Source: three-view drawing plus pictorial views. Frame: mm from the lowest corner of the part. A direction names the side the tool comes from. Coordinates: 2 decimals unless noted, no trailing zeros. Loops run counter-clockwise (first coordinate to the right, second up) from the corner with the lowest first, then second, coordinate; pieces in that order, holes last. Notation, with made-up numbers: M 62.5,-1 L 118.5,-1 A29 cw 118.5,38 Z; hole C -36.5,55 d11. An arc over 180 degrees is marked long. Use a Markdown table: item, result. Add a question column.
1. Pin query (flat end, axial travel): pin 1 (1.8 mm diameter, centred on y = 5.2, z = 63, fed in from +X); pin 2 (3.5 mm diameter, centred on x = 51.3, z = 101.25, fed in from -Y). Return the tip coordinate at first contact, or that it passes through.
2. Section A-A on z = 31.5. Output: boundary loops of the cut face in (x, y) (3 decimals), then the cut area to 3 significant figures.
3. Line query: L1, parallel to X at y = 10.75, z = 32; L2, parallel to X at y = 11.3, z = 123.25; L3, parallel to X at y = 3.5, z = 12 (3 decimals). Output: solid intervals per line, ascending. Write a range as [from, to].
4. Section D-D on z = 93.5. Output: boundary loops of the cut face in (x, y) (3 decimals).
5. Section B-B on x = 23. Output: boundary loops of the cut face in (y, z).
6. Set-up query: the marked faces 1 and 2. Return all of +Z, -Z, +X, -X, +Y, -Y with unobstructed straight access to the full face (end or side cutting, diameter ignored); none if empty.
7. Section C-C on z = 49. Output: boundary loops of the cut face in (x, y) (3 decimals).
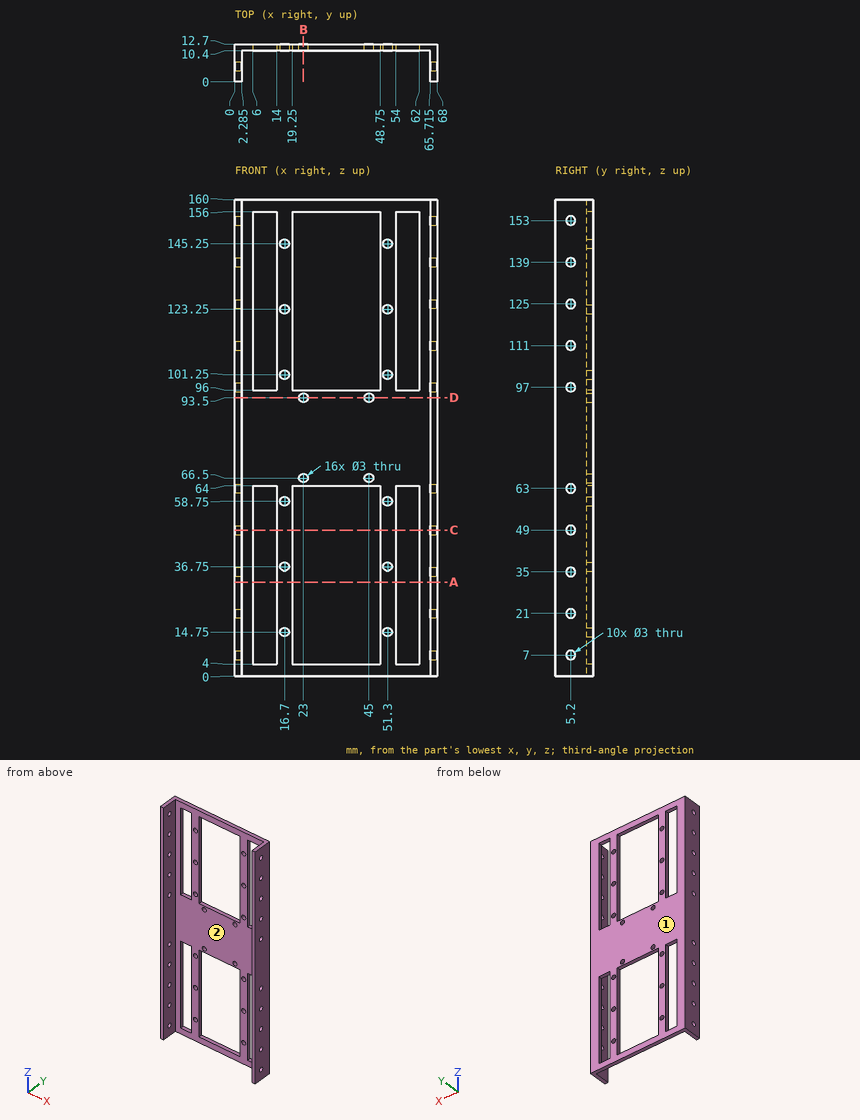
Answers below:
| question | item | result |
|---|---|---|
| 1 | pin 1 | passes through |
| 1 | pin 2 | stops at y = 10.4 |
| 2 | outline | M 0,0 L 2.285,0 L 2.285,10.4 L 6,10.4 L 6,12.7 L 0,12.7 Z; M 14,10.4 L 19.25,10.4 L 19.25,12.7 L 14,12.7 Z; M 48.75,10.4 L 54,10.4 L 54,12.7 L 48.75,12.7 Z; M 62,10.4 L 65.715,10.4 L 65.715,0 L 68,0 L 68,12.7 L 62,12.7 Z |
| 2 | area | 99.3 mm² |
| 3 | L1 | x = [0, 6], [14, 19.25], [48.75, 54], [62, 68] |
| 3 | L2 | x = [0, 6], [14, 15.2], [18.2, 19.25], [48.75, 49.8], [52.8, 54], [62, 68] |
| 3 | L3 | x = [0, 2.285], [65.715, 68] |
| 4 | outline | M 0,0 L 2.285,0 L 2.285,10.4 L 21.5,10.4 L 21.5,12.7 L 0,12.7 Z; M 24.5,10.4 L 43.5,10.4 L 43.5,12.7 L 24.5,12.7 Z; M 46.5,10.4 L 65.715,10.4 L 65.715,0 L 68,0 L 68,12.7 L 46.5,12.7 Z |
| 5 | outline | M 10.4,0 L 12.7,0 L 12.7,4 L 10.4,4 Z; M 10.4,64 L 12.7,64 L 12.7,65 L 10.4,65 Z; M 10.4,68 L 12.7,68 L 12.7,92 L 10.4,92 Z; M 10.4,95 L 12.7,95 L 12.7,96 L 10.4,96 Z; M 10.4,156 L 12.7,156 L 12.7,160 L 10.4,160 Z |
| 6 | face 1 | +Z, -Z, +X, -X, +Y |
| 6 | face 2 | +Z, -Z, -Y |
| 7 | outline | M 0,0 L 2.285,0 L 2.285,3.7 L 0,3.7 Z; M 0,6.7 L 2.285,6.7 L 2.285,10.4 L 6,10.4 L 6,12.7 L 0,12.7 Z; M 14,10.4 L 19.25,10.4 L 19.25,12.7 L 14,12.7 Z; M 48.75,10.4 L 54,10.4 L 54,12.7 L 48.75,12.7 Z; M 62,10.4 L 65.715,10.4 L 65.715,6.7 L 68,6.7 L 68,12.7 L 62,12.7 Z; M 65.715,0 L 68,0 L 68,3.7 L 65.715,3.7 Z |
